Geometry: final body of the model. Coordinates: model frame, mm. Round coordinates to 2 decimals unless told otherwise and drop trailing zeros. Loops run counter-clockwise (first coordinate to the right, second up) from the corner with the lowest first, then second, coordinate; pieces in that order, holes last. Notation, with made-up numbers: (67, 21.5) -> (99, 21.5) arc R13 cw to (99, 39.5) -> close; hole circle Ø2 at (-31.75, 10). An arc over 180 degrees is marked (long way). Answer in a Markdown table with one row per item.
Autodesk Inventor part; units mm, degrees
ref_plane "Work Plane2" through (0, 0, 218.4976) normal (0, 0, 1) x (1, 0, 0)
ref_plane "Work Plane1" through (0, 6.35, 0) normal (0, 1, 0) x (-1, 0, 0)
ref_plane "YZ Plane" through (0, 0, 0) normal (1, 0, 0) x (0, 1, 0)
sketch "Sketch1" plane through (0, 0, 0) normal (0, 0, 1) x (1, 0, 0)
  circle A0 centre (0, 0) radius 6.35
  dimension "d0" = 12.7
extrude "Extrusion1" add sketch "Sketch1" along normal blind 225
ref_plane "Work Plane2" through (0, 0, 218.4976) normal (0, 0, 1) x (1, 0, 0)
sketch "Sketch2" plane through (0, 0, 218.4976) normal (0, 0, 1) x (1, 0, 0)
  circle A0 centre (0, 0) radius 6.35
  line L0 (-5.4993, -3.175) -> (5.4993, -3.175)
  dimension "d3" = 9.525
extrude "Extrusion3" cut sketch "Sketch2" against normal blind 12.7762 contours L0 A0 picked at (-1.5396, -3.5692)
sketch "Sketch3" plane through (-5.4993, -3.175, 218.4976) normal (0, -1, 0) x (1, 0, 0)
  line L0 (0, 0) -> (10.9985, 0)
  line L1 (10.9985, -12.7762) -> (0, -12.7762)
  line L2 (10.9985, 0) -> (10.9985, -12.7762)
  line L3 (10.9985, 0) -> (0, 0)
  line L4 (0, -12.7762) -> (0, 0)
  point P0 (5.4993, -7.9756)
  dimension "d6" = 7.9756
hole "Hole1" at (0, -3.175, 210.522) direction (0, 1, 0) diameter 5.2578 end through all
ref_plane "Work Plane1" through (0, 6.35, 0) normal (0, 1, 0) x (-1, 0, 0)
sketch "Sketch4" plane through (0, 6.35, 0) normal (0, 1, 0) x (-1, 0, 0)
  line L0 (-6.35, 0) -> (6.35, 0)
  point P0 (0, 8.5)
  point P1 (0, 33.9)
  point P2 (0, 210.522)
  dimension "d14" = 25.4
  dimension "d28" = 8.5
hole "Hole2" at (0, 6.35, 8.5) at (0, 6.35, 33.9) direction (0, -1, 0) diameter 6.35 end through all counterbore diameter 12.7 counterbore depth 1.5875
properties part number "PWTR-0031" material "Stainless Steel, 303"
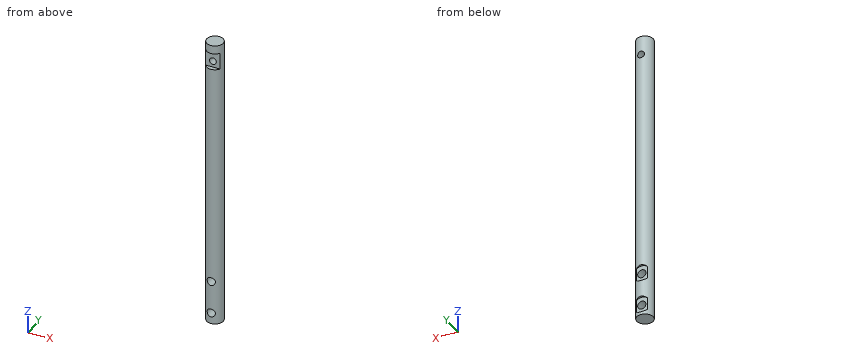
Item 1: Cut plane B-B (y = 0). Output: boundary loops of the cut face in (x, z) (3 decimals), then the cut area to 3 significant figures.
Answer:
| item | result |
|---|---|
| outline | (-6.35, 0) -> (6.35, 0) -> (6.35, 225) -> (-6.35, 225) -> close; hole circle Ø6.35 at (0, 8.5); hole circle Ø6.35 at (0, 33.9); hole circle Ø5.258 at (0, 210.522) |
| area | 2,770 mm² |
Item 2: Cut plane A-A (x = 0). Count the separate pieces of the cut face and the enclosed holes in it, then the cut area to 3 significant figures.
Answer:
| item | result |
|---|---|
| separate pieces | 4 |
| enclosed holes | 0 |
| area | 2,590 mm² |
Item 3: Cut plane D-D (z = 139). Output: boundary loops of the cut face in (x, y), then the cut area to 3 significant figures.
Answer:
| item | result |
|---|---|
| outline | circle Ø12.7 at (0, 0) |
| area | 127 mm² |
Item 4: Line query: probe 1 along Z at (x, y) = (0, 0.75) (3 decimals); probe 2 along Z at (x, y) = (2.25, 5.5); probe 3 along Z at (x, y) = (3.75, -3.25). Output: solid intervals per line, ascending. Write a range as [from, to].
Answer:
| item | result |
|---|---|
| probe 1 | z = [0, 5.325], [11.675, 30.725], [37.075, 207.893], [213.151, 225] |
| probe 2 | z = [0, 2.56], [14.44, 27.96], [39.84, 209.16], [211.88, 225] |
| probe 3 | z = [0, 205.72], [218.5, 225] |
Item 5: Pin query (flat end, axial travel): pin 1 Ø4 at (x, z) = (0, 210.522) entering from +Y (1 decimal); pin 2 Ø6 at (x, y) = (2, 1.5) entering from -Z; pin 3 Ø3.5 at (x, z) = (1.5, 209.5) entering from -Y (3 decimals); pin 4 Ø5 at (x, z) = (-4.5, 81) entering from +Y. Return the tip coordinate at first contact, or that it passes through.
Answer:
| item | result |
|---|---|
| pin 1 | passes through |
| pin 2 | stops at z = 0 |
| pin 3 | stops at y = -3.175 |
| pin 4 | stops at y = 6.03 |
